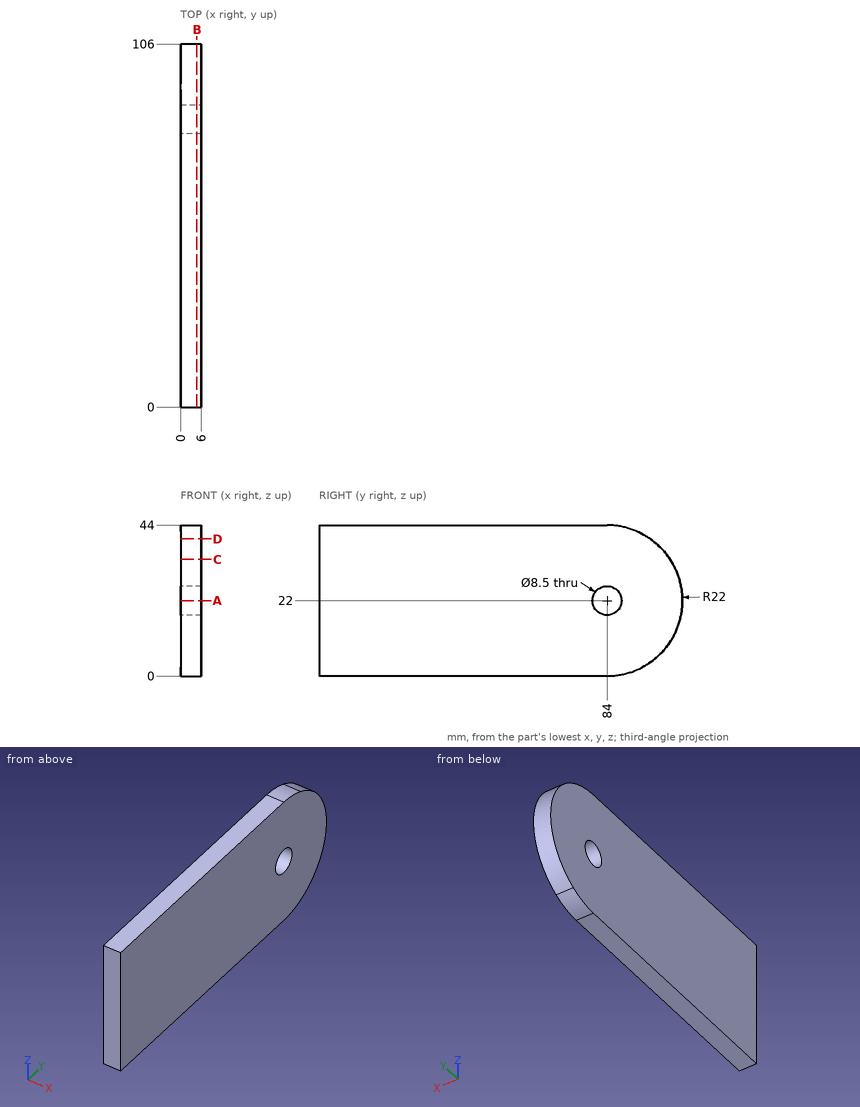
Here's the drawing with two shaded views (mm, measured from the low corner). I have some questions. Round coordinates to 2 decimals unless told otherwise and drop trailing zeros. Loops run counter-clockwise (first coordinate to the right, second up) from the corner with the lowest first, then second, coordinate; pieces in that order, holes last. Notation, with made-up numbers: M 16.5,65 L 54.5,65 A10 ccw 54.5,76 Z; hole C -7,-18 d5. An arc over 180 degrees is marked long. Answer as a JSON object with one key per item and string values. Group by question number.
Q1. Please list where these lines run through material, in increasing order: L1, parallel to Z at x = 2.95, y = 84; L2, parallel to Y at x = 3.95, z = 22; L3, parallel to Z at x = 4.4, y = 81.
Q2. Will these pins go through, and if not, where does the flat tip stop? pin 1 (3 mm diameter, centred on x = 2, z = 14.5, fed in from +Y); pin 2 (7 mm diameter, centred on y = 84, z = 22, fed in from +X).
Q3. Imagine slicing it at B-B, the plane x = 4.75. Please give me the cut outline in (y, z), then the cut area to 3 significant figures.
Q4. Imagine slicing it at D-D, the plane z = 40. Please give me the cut outline in (x, y), then the cut area to 3 significant figures.
Q5. Imagine slicing it at A-A, the plane z = 22. Please give me the cut outline in (x, y), then the cut area to 3 significant figures.
Q6. Imagine slicing it at C-C, the plane z = 34. Please give me the cut outline in (x, y).
Findings:
{
 "1": {"L1": "z = 0 to 17.75, 26.25 to 44", "L2": "y = 0 to 79.75, 88.25 to 106", "L3": "z = 0 to 18.99, 25.01 to 44"},
 "2": {"pin 1": "stops at y = 105.17", "pin 2": "passes through"},
 "3": {"outline": "M 0,0 L 84,0 A22 ccw 94.35,2.59 A22 ccw 92.62,42.24 A22 ccw 84,44 L 0,44 Z; hole C 84,22 d8.5", "area": "4,400 mm2"},
 "4": {"outline": "M 0,0 L 6,0 L 6,96.65 L 0,96.65 Z", "area": "580 mm2"},
 "5": {"outline": "M 0,0 L 6,0 L 6,79.75 L 0,79.75 Z; M 0,88.25 L 6,88.25 L 6,106 L 0,106 Z", "area": "585 mm2"},
 "6": {"outline": "M 0,0 L 6,0 L 6,102.44 L 0,102.44 Z"}
}
